from build123d import *

# Parameters (mm, degrees)
F3_W          = 15.6
F3_H          = 15.6
F4_DEPTH      = 8
F4_DEPTH_BACK = 8
F5_R          = 2
F7_R          = 1.5
F8_DEPTH      = 2.5
F10_R         = 1.5
F11_DEPTH     = 0.4166666667
F13_R         = 1.5
F14_DEPTH     = 1.25
F16_R         = 1.5
F17_DEPTH     = 0.8333333333
F19_R         = 1.5
F20_DEPTH     = 0.625
F22_R         = 1.5
F23_DEPTH     = 0.5


with BuildPart() as f4:
    # F3 (on Top) → F4 (new body, two sides)
    with BuildSketch(Plane.XY) as f4_sk:
        Rectangle(F3_W, F3_H)
    extrude(amount=F4_DEPTH)
    extrude(f4_sk.sketch, amount=-F4_DEPTH_BACK)

    # F5
    f5_edges = [f4.edges().sort_by_distance(p)[0] for p in [
        (0, -7.8, 8),
        (7.8, 0, 8),
        (0, 7.8, 8),
        (-7.8, 0, 8),
        (-7.8, 7.8, 0),
        (7.8, 7.8, 0),
        (0, 7.8, -8),
        (-7.8, 0, -8),
        (7.8, 0, -8),
        (7.8, -7.8, 0),
        (0, -7.8, -8),
        (-7.8, -7.8, 0),
    ]]
    fillet(f5_edges, radius=F5_R)

    # F7 (on offset) → F8 (cut)
    with BuildSketch(Plane(origin=(0, 0, -8), x_dir=(1, 0, 0), z_dir=(0, 0, -1))):
        Circle(F7_R)
    extrude(amount=-F8_DEPTH, mode=Mode.SUBTRACT)

    # F10 (on offset) → F11 (cut)
    with BuildSketch(Plane.XY.offset(8)):
        with Locations((-2, 3.4641016151)):
            Circle(F10_R)
        with Locations((2, 3.4641016151)):
            Circle(F10_R)
        with Locations((4, 0)):
            Circle(F10_R)
        with Locations((2, -3.4641016151)):
            Circle(F10_R)
        with Locations((-2, -3.4641016151)):
            Circle(F10_R)
        with Locations((-4, 0)):
            Circle(F10_R)
    extrude(amount=-F11_DEPTH, mode=Mode.SUBTRACT)

    # F13 (on offset) → F14 (cut)
    with BuildSketch(Plane.XZ.offset(7.8)):
        with Locations((-4, 0)):
            Circle(F13_R)
        with Locations((4, 0)):
            Circle(F13_R)
    extrude(amount=-F14_DEPTH, mode=Mode.SUBTRACT)

    # F16 (on offset) → F17 (cut)
    with BuildSketch(Plane(origin=(-7.8, 0, 0), x_dir=(0, -1, 0), z_dir=(-1, 0, 0))):
        with Locations((-2, 3.4641016151)):
            Circle(F16_R)
        with Locations((-2, -3.4641016151)):
            Circle(F16_R)
        with Locations((4, 0)):
            Circle(F16_R)
    extrude(amount=-F17_DEPTH, mode=Mode.SUBTRACT)

    # F19 (on offset) → F20 (cut)
    with BuildSketch(Plane.YZ.offset(7.8)):
        with Locations((-4, 0)):
            Circle(F19_R)
        with Locations((0, 4)):
            Circle(F19_R)
        with Locations((4, 0)):
            Circle(F19_R)
        with Locations((0, -4)):
            Circle(F19_R)
    extrude(amount=-F20_DEPTH, mode=Mode.SUBTRACT)

    # F22 (on offset) → F23 (cut)
    with BuildSketch(Plane(origin=(0, 7.8, 0), x_dir=(-1, 0, 0), z_dir=(0, 1, 0))):
        with Locations((-3.2360679775, 2.3511410092)):
            Circle(F22_R)
        with Locations((1.2360679775, 3.8042260652)):
            Circle(F22_R)
        with Locations((4, 0)):
            Circle(F22_R)
        with Locations((1.2360679775, -3.8042260652)):
            Circle(F22_R)
        with Locations((-3.2360679775, -2.3511410092)):
            Circle(F22_R)
    extrude(amount=-F23_DEPTH, mode=Mode.SUBTRACT)


solid = f4.part
CAD build for the part. Positions are in the model's coordinates, mm. A direction names the side the tool comes from. Give positions to 0.01 mm unless a question says otherwise; leave off trailing zeros. Write each loop counter-clockwise with the first axis right and the second up, starting at its lowest first coordinate (ties: lowest second). Pieces come first, ordered by that corner, then holes. Notation, with made-up numbers: M 46.5,62 L 75.5,62 A16 ccw 75.5,93 Z; hole C -31.75,65 d4. An arc over 180 degrees is marked long. Put each result on its own line as item: value. Start each with the question number.
(1) Which spindle directions (+Z, -Z, +X, -X, +Y, -Y) get a long thin tool onto all of the face, cutting with end or side? Do faces 5 (the face through (-4, 0, 7.583)), 6 (the face through (-2.614, -7.184, -0.575)), 7 (the face through (-6.967, -4, 0)), 8 (the face through (-0.91, 7.55, -5.27)). Say none if no direction does.
(2) Band-saw the part on B-B, the plane z = 4.25. Write the cut outline in (x, y) (3 decimals).
(3) Mould opens along Y. For faces 1 (the face through (7.492, -0.195, -2.513)), 2 (the face through (7.492, 0.806, 5.265)), 3 (the face through (3, 7.3, -2)), 4 (the face through (-7.23, 0.08, -7.4)) say: +Y half, -Y half, draft (parallel to the pull), parting line (faces both ways), or undercut.
(4) Band-saw the part on A-A, the plane x = -4. Write the cut outline in (y, z), and give its area (3 significant figures).
(5) Band-saw the part on D-D, the plane x = -0.75. Write the cut outline in (y, z).
(6) Probe L1, parallel to Z at x = 7.25, y = 0; L2, parallel to Z at x = 7.5, y = 0; L3, parallel to X at y = 3.25, z = 3.5. List the from-to ranges inside material, lowest first.
(7) Band-saw the part on C-C, the plane y = 6.5. Write the cut outline in (x, z), and give its area (3 significant figures).
(8) Flat gauge pins, fed straight in: pin 1 Ø2.5 at (x, z) = (-1.24, 3.8) entering from +Y; pin 2 Ø0.9 at (x, y) = (1.5, -4) entering from +Z; pin 3 Ø2.5 at (y, z) = (2, -3.46) entering from -X. Where does each tip first touch, or does it go through?
Response values:
1. face 5: +Z
1. face 6: -Y
1. face 7: -X
1. face 8: +Y
2. outline: M -7.8,-5.8 A2 ccw -5.8,-7.8 L 5.8,-7.8 A2 ccw 7.8,-5.8 L 7.8,-1.479 L 7.175,-1.479 L 7.175,1.479 L 7.8,1.479 L 7.8,5.8 A2 ccw 5.8,7.8 L 0.196,7.8 L 0.196,7.3 L -2.668,7.3 L -2.668,7.8 L -5.8,7.8 A2 ccw -7.8,5.8 L -7.8,3.278 L -6.967,3.278 L -6.967,0.722 L -7.8,0.722 Z
3. face 1: undercut
3. face 2: undercut
3. face 3: +Y half
3. face 4: draft
4. outline: M -7.8,-6 A2 ccw -5.8,-8 L 5.8,-8 A2 ccw 7.8,-6 L 7.8,-1.5 L 7.3,-1.5 L 7.3,1.5 L 7.8,1.5 L 7.8,6 A2 ccw 5.8,8 L 1.5,8 L 1.5,7.58 L -1.5,7.58 L -1.5,8 L -5.8,8 A2 ccw -7.8,6 L -7.8,1.5 L -6.55,1.5 L -6.55,-1.5 L -7.8,-1.5 Z
4. area: 240 mm2
5. outline: M -7.8,-6 A2 ccw -5.8,-8 L -1.3,-8 L -1.3,-5.5 L 1.3,-5.5 L 1.3,-8 L 5.8,-8 A2 ccw 7.8,-6 L 7.8,-5.22 L 7.3,-5.22 L 7.3,-2.39 L 7.8,-2.39 L 7.8,2.39 L 7.3,2.39 L 7.3,5.22 L 7.8,5.22 L 7.8,6 A2 ccw 5.8,8 L 4.29,8 L 4.29,7.58 L 2.63,7.58 L 2.63,8 L -2.63,8 L -2.63,7.58 L -4.29,7.58 L -4.29,8 L -5.8,8 A2 ccw -7.8,6 Z
6. L1: z = -7.38 to -5.5, -2.5 to 2.5, 5.5 to 7.38
6. L2: z = -7.05 to -5.5, -2.5 to 2.5, 5.5 to 7.05
6. L3: x = -6.97 to 7.8
7. outline: M -7.67,-6 A1.87 ccw -5.8,-7.87 L 5.8,-7.87 A1.87 ccw 7.67,-6 L 7.67,6 A1.87 ccw 5.8,7.87 L -5.8,7.87 A1.87 ccw -7.67,6 Z
7. area: 239 mm2
8. pin 1: stops at y = 7.3
8. pin 2: stops at z = 7.58
8. pin 3: stops at x = -6.97
